```python
from build123d import *

# Parameters (mm, degrees)
SKETCH1_W          = 300
SKETCH1_H          = 2
BASE_FLANGE1_DEPTH = 352
CHAMFER1_SIZE      = 5
CHAMFER2_SIZE      = 50
CUT_EXTRUDE1_REACH = 384.633
SKETCH2_R          = 2.25
SKETCH3_W          = 40
SKETCH3_H          = 20
CUT_EXTRUDE2_DEPTH = 383.632983419
FILLET1_R          = 10
CHAMFER3_SIZE      = 5


# Sheet-metal steps are written as plain solids
with BuildPart() as part:
    # Sketch1 → Base-Flange1 (new body)
    with BuildSketch(Plane.XY):
        with Locations((0, -1)):
            Rectangle(SKETCH1_W, SKETCH1_H)
    extrude(amount=BASE_FLANGE1_DEPTH)

    # Chamfer1
    chamfer1_edges = [part.edges().sort_by_distance(p)[0] for p in [
        (150, -1, 0),
        (150, -1, 352),
    ]]
    chamfer(chamfer1_edges, length=CHAMFER1_SIZE)

    # Chamfer2
    chamfer2_edges = [part.edges().sort_by_distance(p)[0] for p in [
        (-150, -1, 352),
        (-150, -1, 0),
    ]]
    chamfer(chamfer2_edges, length=CHAMFER2_SIZE)

    # Sketch2 → Cut-Extrude1 (cut, up to next)
    with BuildSketch(Plane.XZ.offset(2), mode=Mode.PRIVATE) as cut_extrude1_sk1:
        with Locations(Location((-37.5, 346, 0), (0, 0, 270))):
            Circle(SKETCH2_R)
    cut_extrude1_tool1 = extrude(cut_extrude1_sk1.sketch, amount=-CUT_EXTRUDE1_REACH, mode=Mode.PRIVATE) & part.part
    # Sketch2 → Cut-Extrude1 (cut, up to next)
    with BuildSketch(Plane.XZ.offset(2), mode=Mode.PRIVATE) as cut_extrude1_sk2:
        with Locations(Location((87.5, 346, 0), (0, 0, 270))):
            Circle(SKETCH2_R)
    cut_extrude1_tool2 = extrude(cut_extrude1_sk2.sketch, amount=-CUT_EXTRUDE1_REACH, mode=Mode.PRIVATE) & part.part
    # Sketch2 → Cut-Extrude1 (cut, up to next)
    with BuildSketch(Plane.XZ.offset(2), mode=Mode.PRIVATE) as cut_extrude1_sk3:
        with Locations(Location((87.5, 6, 0), (0, 0, 270))):
            Circle(SKETCH2_R)
    cut_extrude1_tool3 = extrude(cut_extrude1_sk3.sketch, amount=-CUT_EXTRUDE1_REACH, mode=Mode.PRIVATE) & part.part
    # Sketch2 → Cut-Extrude1 (cut, up to next)
    with BuildSketch(Plane.XZ.offset(2), mode=Mode.PRIVATE) as cut_extrude1_sk4:
        with Locations(Location((-37.5, 6, 0), (0, 0, 270))):
            Circle(SKETCH2_R)
    cut_extrude1_tool4 = extrude(cut_extrude1_sk4.sketch, amount=-CUT_EXTRUDE1_REACH, mode=Mode.PRIVATE) & part.part
    add(cut_extrude1_tool1.solids().sort_by_distance((-37.5, -2, 346))[0], mode=Mode.SUBTRACT)
    add(cut_extrude1_tool2.solids().sort_by_distance((87.5, -2, 346))[0], mode=Mode.SUBTRACT)
    add(cut_extrude1_tool3.solids().sort_by_distance((87.5, -2, 6))[0], mode=Mode.SUBTRACT)
    add(cut_extrude1_tool4.solids().sort_by_distance((-37.5, -2, 6))[0], mode=Mode.SUBTRACT)

    # Sketch3 → Cut-Extrude2 (cut, through all)
    with BuildSketch(Plane(origin=(0, 0, 0), x_dir=(1, 0, 0), z_dir=(0, 1, 0))):
        with Locations((130, -40)):
            Rectangle(SKETCH3_W, SKETCH3_H)
        with Locations((130, -312)):
            Rectangle(SKETCH3_W, SKETCH3_H)
    extrude(amount=-CUT_EXTRUDE2_DEPTH, mode=Mode.SUBTRACT)

    # Fillet1
    fillet1_edges = [part.edges().sort_by_distance(p)[0] for p in [
        (110, -1, 322),
        (110, -1, 302),
        (110, -1, 50),
        (110, -1, 30),
    ]]
    fillet(fillet1_edges, radius=FILLET1_R - 0.0001)  # a hair under: the kernel refuses the full size

    # Chamfer3
    chamfer3_edges = [part.edges().sort_by_distance(p)[0] for p in [
        (150, -1, 30),
        (150, -1, 50),
        (150, -1, 322),
        (150, -1, 302),
    ]]
    chamfer(chamfer3_edges, length=CHAMFER3_SIZE)


solid = part.part
```
Design review of the part built by this model. Coordinates are the model's own, in mm. A direction names the side the tool comes from. Give positions to 0.01 mm unless a question says otherwise; leave off trailing zeros. Loops run counter-clockwise (first coordinate to the right, second up) from the corner with the lowest first, then second, coordinate; pieces in that order, holes last. Notation, with made-up numbers: M 59,32.25 L 76,32.25 A18 cw 76,67.25 Z; hole C 82.25,-27.5 d7. An arc over 180 degrees is marked long. Return JSON: item names as keys, results as strings. Group by question number.
Item 1: Tool access review of faces 4 (the flat face through (-125, -1, 25)), 5 (the cylindrical face through (112.85, -1.01, 46.99)): name each direction out of +Z, -Z, +X, -X, +Y, -Y from which nothing blocks a thin tool from reaching the whole face with its end or side.
Item 2: We need section A-A (y = -0.9). Give the number of separate pieces and of enclosed holes in the cut face, and give its area (3 significant figures).
Item 3: We need section B-B (z = 331.5). Give the boundary of the cut face in (x, y).
Item 4: Insertion check: pin 1 Ø2.5 at (x, z) = (87.5, 346) entering from +Y. The pin has a flat end and moves straight along its axis. Give the tip position at first contact, or say it passes through.
Item 5: Mouldability with a two-part tool opening along Z and no side actions: class faces 1 (the cylindrical face through (113.01, -1.01, 304.85)), 2 (the flat face through (-125, -1, 327)), 3 (the flat face through (-2, 0, 174)) as released by +Z, released by -Z, zero draft, split by the parting line, or undercut.
Item 6: For probe 1 along Z at (x, y) = (122, -0.2); probe 2 along X at (y, z) = (-0.5, 346); probe 3 along Z at (x, y) = (-129, -0.45), list the stretches that pass through material, from the lowest coordinate up.
Output:
{
 "1": {"face 4": "-Z, -X, +Y, -Y", "face 5": "+X, +Y, -Y"},
 "2": {"separate pieces": "1", "enclosed holes": "4", "area": "101,000 mm^2"},
 "3": {"outline": "M -120.5,-2 L 150,-2 L 150,0 L -120.5,0 Z"},
 "4": {"pin 1": "passes through"},
 "5": {"face 1": "undercut", "face 2": "released by +Z", "face 3": "zero draft"},
 "6": {"probe 1": "z = 0 to 30, 50 to 302, 322 to 352", "probe 2": "x = -106 to -39.75, -35.25 to 85.25, 89.75 to 150", "probe 3": "z = 29 to 323"}
}
